Design review of the part built by this model. Coordinates are the model's own, in mm. A direction names the side the tool comes from. Give positions to 0.01 mm unless a question says otherwise; leave off trailing zeros. Order: outer loops, then holes, each group sorted by start corner. A loop starts at its lowest first (then second) coordinate and runs counter-clockwise, first axis right, second up. Notation, with made-up numbers: M 58.25,46.5 L 78.25,46.5 A26 cw 78.25,69.5 Z; hole C 69.5,-32 d1. An arc over 180 degrees is marked long. Answer as a JSON object with one key per item and string values.
from build123d import *

# Parameters (mm, degrees)
F1_DEPTH = 609.6
F3_DEPTH = 50.801


with BuildPart() as f1:
    # F0 (on Front) → F1 (new body)
    with BuildSketch(Plane.XZ):
        with BuildLine():
            Line((-18.9612670034, -25.2729933709), (19.1387329966, -25.2729933709))
            ThreePointArc((19.1387329966, -25.2729933709), (23.6288610571, -23.4131214314), (25.4887329966, -18.9229933709))
            Line((25.4887329966, -18.9229933709), (25.4887329966, 19.1770066291))
            ThreePointArc((25.4887329966, 19.1770066291), (23.6288610571, 23.6671346896), (19.1387329966, 25.5270066291))
            Line((19.1387329966, 25.5270066291), (-18.9612670034, 25.5270066291))
            ThreePointArc((-18.9612670034, 25.5270066291), (-23.451395064, 23.6671346896), (-25.3112670034, 19.1770066291))
            Line((-25.3112670034, 19.1770066291), (-25.3112670034, -18.9229933709))
            ThreePointArc((-25.3112670034, -18.9229933709), (-23.451395064, -23.4131214314), (-18.9612670034, -25.2729933709))
        make_face()
        with BuildLine():
            Line((-18.9612670034, 22.3520066291), (19.1387329966, 22.3520066291))
            ThreePointArc((19.1387329966, 22.3520066291), (21.3837970268, 21.4220706594), (22.3137329966, 19.1770066291))
            Line((22.3137329966, 19.1770066291), (22.3137329966, -18.9229933709))
            ThreePointArc((22.3137329966, -18.9229933709), (21.3837970268, -21.1680574012), (19.1387329966, -22.0979933709))
            Line((19.1387329966, -22.0979933709), (-18.9612670034, -22.0979933709))
            ThreePointArc((-18.9612670034, -22.0979933709), (-21.2063310337, -21.1680574012), (-22.1362670034, -18.9229933709))
            Line((-22.1362670034, -18.9229933709), (-22.1362670034, 19.1770066291))
            ThreePointArc((-22.1362670034, 19.1770066291), (-21.2063310337, 21.4220706594), (-18.9612670034, 22.3520066291))
        make_face(mode=Mode.SUBTRACT)
    extrude(amount=F1_DEPTH)

    # F2 (on face) → F3 (cut, through all)
    with BuildSketch(Plane.YZ.offset(25.4887329966)):
        Polygon((-637.5276456785, 54.5883400366), (-637.5276456785, -53.2560676181), (-603.1945714313, -18.9229933709), (-609.6, -18.9229933709), (-609.6, 19.1770066291), (-565.0945714313, 19.1770066291), (-529.6832380238, 54.5883400366), align=None)
        Polygon((-609.6, -18.9229933709), (-603.1945714313, -18.9229933709), (-565.0945714313, 19.1770066291), (-609.6, 19.1770066291), align=None)
        Polygon((0, -18.9229933709), (-5.9980263665, -18.9229933709), (48.8678000444, -73.7888197817), (48.8678000444, 69.9899916479), (-94.9110113853, 69.9899916479), (-44.0980263665, 19.1770066291), (0, 19.1770066291), align=None)
        Polygon((-44.0980263665, 19.1770066291), (-5.9980263665, -18.9229933709), (0, -18.9229933709), (0, 19.1770066291), align=None)
    extrude(amount=-F3_DEPTH, mode=Mode.SUBTRACT)


solid = f1.part
(1) To check wall thickness, follow L1, parallel to Z at x = 8.5, y = -534; L2, parallel to X at y = -150.5, z = 16; L3, parallel to Z at x = 20, y = -190. State the ranges of each line that lie inside material, in increasing order. Write a range as from..to.
Checked values:
{"L1": "z = -25.27..-22.1, 22.35..25.53", "L2": "x = -25.31..-22.14, 22.31..25.49", "L3": "z = -25.21..-21.98, 22.23..25.47"}
(2) Draft analysis for pull direction X (two halves, no side actions). For faces 1 (the flat face through (-22.136, -300, 0)), 2 (the flat face through (0, -301, 25.527)), 3 (the flat face through (0, -301, 22.352)), 4 (the flat face through (-25.311, -300, 0)), state which applies: +X half, -X half, draft (parallel to the pull), parting line (faces both ways), or undercut.
Checked values:
{"face 1": "undercut", "face 2": "draft", "face 3": "undercut", "face 4": "-X half"}
(3) We need section B-B (z = -10.5). Write out the cut boundary in (x, y).
Checked values:
{"outline": "M -25.31,-594.77 L -22.14,-594.77 L -22.14,-14.42 L -25.31,-14.42 Z; M 22.31,-594.77 L 25.49,-594.77 L 25.49,-14.42 L 22.31,-14.42 Z"}
(4) Tool access review of faces 5 (the flat face through (22.314, -300, 0)), 6 (the flat face through (-22.37, -584.26, 0.01)): name each direction out of +Z, -Z, +X, -X, +Y, -Y from which nothing blocks a thin tool from reaching the whole face with its end or side.
Checked values:
{"face 5": "+Y, -Y", "face 6": "+Z, +X, -X, -Y"}
(5) We need section D-D (y = -572). Write out the cut boundary in (x, z) (3 decimals).
Checked values:
{"outline": "M -25.311,-18.923 A6.35 ccw -18.961,-25.273 L 19.139,-25.273 A6.35 ccw 25.489,-18.923 L 25.489,12.272 L 22.314,12.272 L 22.314,-18.923 A3.175 cw 19.139,-22.098 L -18.961,-22.098 A3.175 cw -22.136,-18.923 L -22.136,12.272 L -25.311,12.272 Z"}
(6) We need section A-A (x = -10.5). Write out the cut boundary in (y, z).
Checked values:
{"outline": "M -609.54,-25.27 L 0,-25.27 L 0,-24.92 L -2.82,-22.1 L -606.37,-22.1 Z; M -561.92,22.35 L -47.27,22.35 L -50.45,25.53 L -558.74,25.53 Z"}
(7) We need section C-C (y = -73). Write out the cut boundary in (x, z) (3 decimals), plus the area to 3 significant figures.
Checked values:
{"outline": "M -25.311,-18.923 A6.35 ccw -18.961,-25.273 L 19.139,-25.273 A6.35 ccw 25.489,-18.923 L 25.489,19.177 A6.35 ccw 19.139,25.527 L -18.961,25.527 A6.35 ccw -25.311,19.177 Z; hole M -22.136,-18.923 A3.175 ccw -18.961,-22.098 L 19.139,-22.098 A3.175 ccw 22.314,-18.923 L 22.314,19.177 A3.175 ccw 19.139,22.352 L -18.961,22.352 A3.175 ccw -22.136,19.177 Z", "area": "579 mm^2"}
